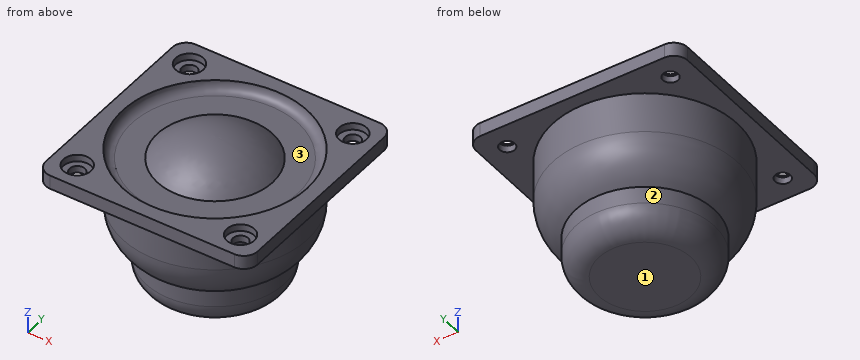
```python
from build123d import *

# Parameters (mm, degrees)
ESQUISSE1_R             = 1.65
BOSS_EXTRU_1_DEPTH      = 3
ESQUISSE2_R             = 3
ENL_V_MAT_EXTRU_1_DEPTH = 1.5
ESQUISSE3_R             = 20
BOSS_EXTRU_2_DEPTH      = 17.4
ESQUISSE4_R             = 15
BOSS_EXTRU_3_DEPTH      = 8.7
CONG_1_R                = 10
CONG_2_R                = 5
ESQUISSE5_R             = 20
ENL_V_MAT_EXTRU_2_DEPTH = 2
ESQUISSE6_R             = 12.5
BOSS_EXTRU_4_DEPTH      = 5
CONG_3_R                = 18
CONG_4_R                = 2


# Some blends are built 0.0001 mm under size
with BuildPart() as part:
    # Esquisse1 → Boss.-Extru.1 (new body)
    with BuildSketch(Plane.XY):
        with BuildLine():
            Line((-20, 23), (20, 23))
            ThreePointArc((20, 23), (22.121320344, 22.121320344), (23, 20))
            Line((23, 20), (23, -20))
            ThreePointArc((23, -20), (22.121320344, -22.121320344), (20, -23))
            Line((20, -23), (-20, -23))
            ThreePointArc((-20, -23), (-22.121320344, -22.121320344), (-23, -20))
            Line((-23, -20), (-23, 20))
            ThreePointArc((-23, 20), (-22.121320344, 22.121320344), (-20, 23))
        make_face()
        with Locations((17.748380208, 17.748380208)):
            Circle(ESQUISSE1_R, mode=Mode.SUBTRACT)
        with Locations((-17.748380208, 17.748380208)):
            Circle(ESQUISSE1_R, mode=Mode.SUBTRACT)
        with Locations((17.748380208, -17.748380208)):
            Circle(ESQUISSE1_R, mode=Mode.SUBTRACT)
        with Locations((-17.748380208, -17.748380208)):
            Circle(ESQUISSE1_R, mode=Mode.SUBTRACT)
    extrude(amount=BOSS_EXTRU_1_DEPTH)

    # Esquisse2 → Enlèv. mat.-Extru.1 (cut)
    with BuildSketch(Plane.XY.offset(3)):
        with Locations((-17.748380208, 17.748380208)):
            Circle(ESQUISSE2_R)
        with Locations((17.748380208, 17.748380208)):
            Circle(ESQUISSE2_R)
        with Locations((17.748380208, -17.748380208)):
            Circle(ESQUISSE2_R)
        with Locations((-17.748380208, -17.748380208)):
            Circle(ESQUISSE2_R)
    extrude(amount=-ENL_V_MAT_EXTRU_1_DEPTH, mode=Mode.SUBTRACT)

    # Esquisse3 → Boss.-Extru.2 (add)
    with BuildSketch(Plane(origin=(0, 0, 0), x_dir=(-1, 0, 0), z_dir=(0, 0, -1))):
        with Locations(Location((0, 0, 0), (0, 0, 180))):
            Circle(ESQUISSE3_R)
    extrude(amount=BOSS_EXTRU_2_DEPTH)

    # Esquisse4 → Boss.-Extru.3 (add)
    with BuildSketch(Plane(origin=(0, 0, -17.4), x_dir=(-1, 0, 0), z_dir=(0, 0, -1))):
        Circle(ESQUISSE4_R)
    extrude(amount=BOSS_EXTRU_3_DEPTH)

    # Congé1
    # the kernel refuses this fillet: 10 mm, written as the material it takes off along each edge
    with BuildSketch(Plane(origin=(0, 0, -17.4), x_dir=(1, 0, 0), z_dir=(0, 1, 0))) as cong_1_piece_1_section:
        with BuildLine():
            CenterArc((10, -8.660254038), CONG_1_R, 0, 60)
            Line((15, 0), (15.1, 0.173205081))
            ThreePointArc((15.1, 0.173205081), (17.5, 0.2), (20, 0.2))
            Line((20, 0.2), (20.2, 0))
            Line((20.2, 0), (20.2, -8.660254038))
            Line((20.2, -8.660254038), (20, -8.660254038))
        make_face()
    cong_1_piece_1 = revolve(axis=Axis((0, 0, -17.4), (0, 0, -1)), mode=Mode.PRIVATE)
    cong_1_piece_1 = cong_1_piece_1 - Plane(origin=(0, 0, -13.800562686), x_dir=(-1, 0, 0), z_dir=(0, 0, 1)) * Cylinder(15, 81, mode=Mode.PRIVATE)
    add(cong_1_piece_1, mode=Mode.SUBTRACT)

    # Congé2
    cong_2_edges = [part.edges().sort_by_distance(p)[0] for p in [
        (15, 0, -26.1),
    ]]
    fillet(cong_2_edges, radius=CONG_2_R)

    # Esquisse5 → Enlèv. mat.-Extru.2 (cut)
    with BuildSketch(Plane.XY.offset(3)):
        Circle(ESQUISSE5_R)
    extrude(amount=-ENL_V_MAT_EXTRU_2_DEPTH, mode=Mode.SUBTRACT)

    # Esquisse6 → Boss.-Extru.4 (add)
    with BuildSketch(Plane.XY.offset(1)):
        Circle(ESQUISSE6_R)
    extrude(amount=BOSS_EXTRU_4_DEPTH)

    # Congé3
    # the kernel refuses this fillet: 18 mm, written as the material it takes off along each edge
    with BuildSketch(Plane(origin=(0, 0, 6), x_dir=(1, 0, 0), z_dir=(0, -1, 0))) as cong_3_piece_1:
        with BuildLine():
            CenterArc((0.050100402, -18), CONG_3_R, 46.238257307, 43.761742693)
            Line((0.050100402, 0), (0.050100402, 0.36))
            Line((0.050100402, 0.36), (12.5, 0.36))
            Line((12.5, 0.36), (12.86, 0))
            ThreePointArc((12.86, 0), (12.86, -2.5), (12.748997992, -4.74))
            Line((12.748997992, -4.74), (12.5, -5))
        make_face()
    revolve(axis=Axis((0, 0, 6), (0, 0, 1)), mode=Mode.SUBTRACT)

    # Congé4
    cong_4_edges = [part.edges().sort_by_distance(p)[0] for p in [
        (-20, 0, 1),
    ]]
    fillet(cong_4_edges, radius=CONG_4_R - 0.0001)  # a hair under: the kernel refuses the full size


solid = part.part
```
Check sheet for the modelled part. Datum: model origin and axes. Units: mm. Face numbers are marked on the shaded views. Round coordinates to 2 decimals unless told otherwise and drop trailing zeros. Order: outer loops, then holes, each group sorted by start corner. A loop starts at its lowest first (then second) coordinate and runs counter-clockwise, first axis right, second up.
1) Section check A-A (z = -19). Record the boundary of the cut face in (x, y).
2) Mould release check, pull along Y, two halves, no side actions. Record for the marked faces 1, 2 and 3: +Y half, -Y half, draft (parallel to the pull), parting line (faces both ways), or undercut.
3) Section check B-B (z = -7.5). Record the boundary of the cut face in (x, y).
4) Go/stop test with flat-tipped pins: pin 1 Ø5.5 at (x, y) = (-17.75, 17.75) entering from -Z; pin 2 Ø14 at (x, y) = (-1, -9.5) entering from +Z; pin 3 Ø2 at (x, y) = (-1, -5) entering from +Z. Record where each tip stops, or that it passes through.
5) Scan lines: line 1 (Z direction, x = -16.5, y = -20); line 2 (Y direction, x = -13.5, z = -7.5); line 3 (Y direction, x = -12, z = 2). Record each from-to range of solid material in increasing order.
Result:
1. outline: circle Ø30 at (0, 0)
2. face 1: draft
2. face 2: parting line
2. face 3: undercut
3. outline: circle Ø40 at (0, 0)
4. pin 1: stops at z = 0
4. pin 2: stops at z = 5.83
4. pin 3: stops at z = 5.54
5. line 1: z = 0 to 1.5
5. line 2: y = -14.76 to 14.76
5. line 3: y = -23 to -15.66, 15.66 to 23
